Geometry check sheet. Reference: the model listing, model coordinates, mm. A direction names the side the tool comes from. Coordinates: 2 decimals unless noted, no trailing zeros. Loops run counter-clockwise (first coordinate to the right, second up) from the corner with the lowest first, then second, coordinate; pieces in that order, holes last. Notation, with made-up numbers: (83, -16) -> (89, -16) arc R6 cw to (89, -8) -> close; hole circle Ø1 at (36.25, 1). An arc over 180 degrees is marked (long way). Answer as a JSON object with one key per item and string values.
from build123d import *

# Parameters (mm, degrees)
SKETCH_1_W                = 60
SKETCH_1_H                = 60
SKETCH_1_W_2              = 50
SKETCH_1_H_2              = 50
EXTRUDE_1_DEPTH           = 84
EXTRUDE_2_DEPTH           = 34
EXTRUDE_5_DEPTH           = 34
EXTRUDE_6_DEPTH           = 34
EXTRUDE_7_DEPTH           = 34
SKETCH_12_R               = 36.5
EXTRUDE_8_DEPTH           = 5
EXTRUDE_START             = -5
SKETCH_13_R               = 36.5
EXTRUDE_9_DEPTH           = 5
SKETCH_14_R               = 36.5
EXTRUDE_10_DEPTH          = 5
SKETCH_15_R               = 36.5
EXTRUDE_11_DEPTH          = 5
SKETCH_22_W               = 29
SKETCH_22_H               = 28.5
SKETCH_22_W_2             = 28.5
SKETCH_22_H_2             = 29
EXTRUDE_12_DEPTH          = 60
SKETCH_18_R               = 1.45
CUT_EXTRUDE_2_DEPTH       = 5
PATTERN_CIRCULAR_1_COUNT  = 8
SKETCH_19_R               = 1.45
CUT_EXTRUDE_3_DEPTH       = 5
PATTERN_CIRCULAR_2_COUNT  = 8
CUT_EXTRUDE_START         = -5
SKETCH_20_R               = 1.45
CUT_EXTRUDE_4_DEPTH       = 5
PATTERN_CIRCULAR_3_COUNT  = 8
SKETCH_21_R               = 1.45
CUT_EXTRUDE_5_DEPTH       = 5
PATTERN_CIRCULAR_4_COUNT  = 8
SKETCH_26_W               = 34
SKETCH_26_H               = 28.5
SKETCH_26_W_2             = 28.5
SKETCH_26_H_2             = 34
CUT_EXTRUDE_7_DEPTH       = 58.75
SKETCH_27_R               = 10.5
CUT_EXTRUDE_8_DEPTH       = 200
SKETCH_28_R               = 10.5
CUT_EXTRUDE_9_DEPTH       = 200
SKETCH_31_R               = 2.4
CUT_EXTRUDE_12_DEPTH      = 200
SKETCH_32_R               = 2.4
CUT_EXTRUDE_13_DEPTH      = 200
CUT_EXTRUDE_14_DEPTH      = 50
CUT_EXTRUDE_14_DEPTH_BACK = 40
SKETCH_33_W               = 11
SKETCH_33_H               = 10
CUT_EXTRUDE_15_DEPTH      = 60
CUT_EXTRUDE_15_DEPTH_BACK = 40
SKETCH_34_W               = 10
SKETCH_34_H               = 11
SKETCH_35_W               = 11
SKETCH_35_H               = 10
CUT_EXTRUDE_16_DEPTH      = 80
SKETCH_36_W               = 10
SKETCH_36_H               = 11
CUT_EXTRUDE_17_DEPTH      = 80


with BuildPart() as part:
    # 草图1 → 拉伸-薄壁1 (new body)
    with BuildSketch(Plane.XY):
        with Locations((-65.869565217, 24.858695652)):
            Rectangle(SKETCH_1_W, SKETCH_1_H)
        with Locations((-65.869565217, 24.858695652)):
            Rectangle(SKETCH_1_W_2, SKETCH_1_H_2, mode=Mode.SUBTRACT)
    extrude(amount=EXTRUDE_1_DEPTH)

    # 草图5 → 凸台-拉伸2 (add)
    with BuildSketch(Plane(origin=(-35.869565217, 0, 0), x_dir=(0, 0, -1), z_dir=(1, 0, 0))):
        Polygon((0, 54.858695652), (-5, 54.858695652), (-84, 54.858695652), (-84, 39.108695652), (-5, 39.108695652), (-5, 10.608695652), (-84, 10.608695652), (-84, -5.141304348), (-5, -5.141304348), (0, -5.141304348), align=None)
    extrude(amount=EXTRUDE_2_DEPTH)

    # 草图8 → 凸台-拉伸5 (add)
    with BuildSketch(Plane(origin=(0, 54.858695652, 0), x_dir=(1, 0, 0), z_dir=(0, 1, 0))):
        Polygon((-95.869565217, 0), (-35.869565217, 0), (-35.869565217, -5), (-35.869565217, -84), (-51.619565217, -84), (-51.619565217, -5), (-80.119565217, -5), (-80.119565217, -84), (-95.869565217, -84), (-95.869565217, -5), align=None)
    extrude(amount=EXTRUDE_5_DEPTH)

    # 草图9 → 凸台-拉伸6 (add)
    with BuildSketch(Plane.ZY.offset(95.869565217)):
        Polygon((0, -5.141304348), (5, -5.141304348), (84, -5.141304348), (84, 10.608695652), (5, 10.608695652), (5, 39.108695652), (84, 39.108695652), (84, 54.858695652), (5, 54.858695652), (0, 54.858695652), align=None)
    extrude(amount=EXTRUDE_6_DEPTH)

    # 草图10 → 凸台-拉伸7 (add)
    with BuildSketch(Plane(origin=(0, -5.141304348, 0), x_dir=(-1, 0, 0), z_dir=(0, -1, 0))):
        Polygon((95.869565217, 0), (35.869565217, 0), (35.869565217, -6.658214143), (35.869565217, -84), (51.619565217, -84), (51.619565217, -6.658214143), (80.119565217, -6.658214143), (80.119565217, -84), (95.869565217, -84), (95.869565217, -6.658214143), align=None)
    extrude(amount=EXTRUDE_7_DEPTH)

    # 草图12 → 凸台-拉伸8 (add)
    with BuildSketch(Plane.ZY.offset(129.869565217)):
        with Locations((36.5, 24.858695652)):
            Circle(SKETCH_12_R)
    extrude(amount=-EXTRUDE_8_DEPTH)

    # 草图13 → 凸台-拉伸9 (add)
    with BuildSketch(Plane(origin=(-1.869565217, 0, 0), x_dir=(0, 0, -1), z_dir=(1, 0, 0)).offset(EXTRUDE_START)):
        with Locations((-36.5, 24.858695652)):
            Circle(SKETCH_13_R)
    extrude(amount=EXTRUDE_9_DEPTH)

    # 草图14 → 凸台-拉伸10 (add)
    with BuildSketch(Plane(origin=(0, 88.858695652, 0), x_dir=(1, 0, 0), z_dir=(0, 1, 0))):
        with Locations((-65.869565217, -36.5)):
            Circle(SKETCH_14_R)
    extrude(amount=-EXTRUDE_10_DEPTH)

    # 草图15 → 凸台-拉伸11 (add)
    with BuildSketch(Plane(origin=(0, -39.141304348, 0), x_dir=(-1, 0, 0), z_dir=(0, -1, 0)).offset(EXTRUDE_START)):
        with Locations((65.869565217, -36.5)):
            Circle(SKETCH_15_R)
    extrude(amount=EXTRUDE_11_DEPTH)

    # 草图22 → 凸台-拉伸12 (add)
    with BuildSketch(Plane.XY.offset(5)):
        with Locations((-110.369565217, 24.858695652)):
            Rectangle(SKETCH_22_W, SKETCH_22_H)
        with Locations((-65.869565217, 69.358695652)):
            Rectangle(SKETCH_22_W_2, SKETCH_22_H_2)
        with Locations((-21.369565217, 24.858695652)):
            Rectangle(SKETCH_22_W, SKETCH_22_H)
        with Locations((-65.869565217, -19.641304348)):
            Rectangle(SKETCH_22_W_2, SKETCH_22_H_2)
    extrude(amount=EXTRUDE_12_DEPTH)

    # 草图18 → 切除-拉伸2 (cut)
    with BuildSketch(Plane(origin=(0, 88.858695652, 0), x_dir=(1, 0, 0), z_dir=(0, 1, 0))):
        with Locations(Location((-98.369565217, -36.5, 0), (0, 0, 270))):
            Circle(SKETCH_18_R)
    cut_extrude_2 = extrude(amount=-CUT_EXTRUDE_2_DEPTH, mode=Mode.SUBTRACT)

    # 阵列(圆周)1: 切除-拉伸2 ×8 about axis
    pattern_circular_1_axis = Axis((-65.869565217, 0, 36.5), (0, 1, 0))
    for i in range(1, PATTERN_CIRCULAR_1_COUNT):
        add(cut_extrude_2.rotate(pattern_circular_1_axis, i * 360 / PATTERN_CIRCULAR_1_COUNT), mode=Mode.SUBTRACT)

    # 草图19 → 切除-拉伸3 (cut)
    with BuildSketch(Plane(origin=(-1.869565217, 0, 0), x_dir=(0, 0, -1), z_dir=(1, 0, 0))):
        with Locations(Location((-36.5, 57.358695652, 0), (0, 0, 90))):
            Circle(SKETCH_19_R)
    cut_extrude_3 = extrude(amount=-CUT_EXTRUDE_3_DEPTH, mode=Mode.SUBTRACT)

    # 阵列(圆周)2: 切除-拉伸3 ×8 about axis
    pattern_circular_2_axis = Axis((0, 24.858695652, 36.5), (1, 0, 0))
    for i in range(1, PATTERN_CIRCULAR_2_COUNT):
        add(cut_extrude_3.rotate(pattern_circular_2_axis, i * 360 / PATTERN_CIRCULAR_2_COUNT), mode=Mode.SUBTRACT)

    # 草图20 → 切除-拉伸4 (cut)
    with BuildSketch(Plane(origin=(0, -39.141304348, 0), x_dir=(-1, 0, 0), z_dir=(0, -1, 0)).offset(CUT_EXTRUDE_START)):
        with Locations(Location((98.369565217, -36.5, 0), (0, 0, 270))):
            Circle(SKETCH_20_R)
    cut_extrude_4 = extrude(amount=CUT_EXTRUDE_4_DEPTH, mode=Mode.SUBTRACT)

    # 阵列(圆周)3: 切除-拉伸4 ×8 about axis
    pattern_circular_3_axis = Axis((-65.869565217, 0, 36.5), (0, 1, 0))
    for i in range(1, PATTERN_CIRCULAR_3_COUNT):
        add(cut_extrude_4.rotate(pattern_circular_3_axis, i * 360 / PATTERN_CIRCULAR_3_COUNT), mode=Mode.SUBTRACT)

    # 草图21 → 切除-拉伸5 (cut)
    with BuildSketch(Plane.ZY.offset(129.869565217).offset(CUT_EXTRUDE_START)):
        with Locations(Location((36.5, 57.358695652, 0), (0, 0, 90))):
            Circle(SKETCH_21_R)
    cut_extrude_5 = extrude(amount=CUT_EXTRUDE_5_DEPTH, mode=Mode.SUBTRACT)

    # 阵列(圆周)4: 切除-拉伸5 ×8 about axis
    pattern_circular_4_axis = Axis((0, 24.858695652, 36.5), (1, 0, 0))
    for i in range(1, PATTERN_CIRCULAR_4_COUNT):
        add(cut_extrude_5.rotate(pattern_circular_4_axis, i * 360 / PATTERN_CIRCULAR_4_COUNT), mode=Mode.SUBTRACT)

    # 草图26 → 切除-拉伸7 (cut)
    with BuildSketch(Plane.XY.offset(84)):
        with Locations((-112.869565217, 24.858695652)):
            Rectangle(SKETCH_26_W, SKETCH_26_H)
        with Locations((-65.869565217, 71.858695652)):
            Rectangle(SKETCH_26_W_2, SKETCH_26_H_2)
        with Locations((-18.869565217, 24.858695652)):
            Rectangle(SKETCH_26_W, SKETCH_26_H)
        with Locations((-65.869565217, -22.141304348)):
            Rectangle(SKETCH_26_W_2, SKETCH_26_H_2)
    extrude(amount=-CUT_EXTRUDE_7_DEPTH, mode=Mode.SUBTRACT)

    # 草图27 → 切除-拉伸8 (cut)
    with BuildSketch(Plane.ZY.offset(129.869565217)):
        with Locations((36.5, 24.858695652)):
            Circle(SKETCH_27_R)
    extrude(amount=-CUT_EXTRUDE_8_DEPTH, mode=Mode.SUBTRACT)

    # 草图28 → 切除-拉伸9 (cut)
    with BuildSketch(Plane(origin=(0, 88.858695652, 0), x_dir=(1, 0, 0), z_dir=(0, 1, 0))):
        with Locations(Location((-65.869565217, -36.5, 0), (0, 0, 270))):
            Circle(SKETCH_28_R)
    extrude(amount=-CUT_EXTRUDE_9_DEPTH, mode=Mode.SUBTRACT)

    # 草图31 → 切除-拉伸12 (cut)
    with BuildSketch(Plane.ZY.offset(95.869565217)):
        with Locations((28.5, 13.858695652)):
            Circle(SKETCH_31_R)
        with Locations((28.5, 35.858695652)):
            Circle(SKETCH_31_R)
        with Locations((68.5, 35.858695652)):
            Circle(SKETCH_31_R)
        with Locations((68.5, 13.858695652)):
            Circle(SKETCH_31_R)
    extrude(amount=-CUT_EXTRUDE_12_DEPTH, mode=Mode.SUBTRACT)

    # 草图32 → 切除-拉伸13 (cut)
    with BuildSketch(Plane(origin=(0, -5.141304348, 0), x_dir=(-1, 0, 0), z_dir=(0, -1, 0))):
        with Locations(Location((76.869565217, -28.5, 0), (0, 0, 90))):
            Circle(SKETCH_32_R)
        with Locations(Location((54.869565217, -28.5, 0), (0, 0, 90))):
            Circle(SKETCH_32_R)
        with Locations(Location((54.869565217, -68.5, 0), (0, 0, 90))):
            Circle(SKETCH_32_R)
        with Locations(Location((76.869565217, -68.5, 0), (0, 0, 90))):
            Circle(SKETCH_32_R)
    extrude(amount=-CUT_EXTRUDE_13_DEPTH, mode=Mode.SUBTRACT)

    # 草图33 → 切除-拉伸14 (cut, two sides: drawn at the far end of the back side and taken through both)
    with BuildSketch(Plane.ZY.offset(51.619565217).offset(-CUT_EXTRUDE_14_DEPTH_BACK)):
        with Locations((50.75, -10.141304348)):
            Rectangle(SKETCH_33_W, SKETCH_33_H)
    extrude(amount=CUT_EXTRUDE_14_DEPTH + CUT_EXTRUDE_14_DEPTH_BACK, mode=Mode.SUBTRACT)

    # 草图34 → 切除-拉伸15 (cut, two sides: drawn at the far end of the back side and taken through both)
    with BuildSketch(Plane(origin=(0, 10.608695652, 0), x_dir=(1, 0, 0), z_dir=(0, 1, 0)).offset(-CUT_EXTRUDE_15_DEPTH_BACK)):
        with Locations((-100.869565217, -50.75)):
            Rectangle(SKETCH_34_W, SKETCH_34_H)
    extrude(amount=CUT_EXTRUDE_15_DEPTH + CUT_EXTRUDE_15_DEPTH_BACK, mode=Mode.SUBTRACT)

    # 草图35 → 切除-拉伸16 (cut)
    with BuildSketch(Plane.ZY.offset(95.869565217)):
        with Locations((50.75, 59.858695652)):
            Rectangle(SKETCH_35_W, SKETCH_35_H)
    extrude(amount=-CUT_EXTRUDE_16_DEPTH, mode=Mode.SUBTRACT)

    # 草图36 → 切除-拉伸17 (cut)
    with BuildSketch(Plane(origin=(0, 54.858695652, 0), x_dir=(1, 0, 0), z_dir=(0, 1, 0))):
        with Locations((-30.869565217, -50.75)):
            Rectangle(SKETCH_36_W, SKETCH_36_H)
    extrude(amount=-CUT_EXTRUDE_17_DEPTH, mode=Mode.SUBTRACT)


solid = part.part
1. Depth check by flat-ended pin: P1, Ø2, axis at x = -62, y = 2, coming from the +Z side; P2, Ø8.5, axis at x = -61.5, y = -14.5, coming from the +Z side; P3, Ø1.7, axis at x = -42.89, z = 13.52, coming from the +Y side; P4, Ø1.5, axis at y = -21.5, z = 44.5, coming from the -X side. Enter the tip coordinate at first touch or a pass-through.
Evaluation:
{"P1": "passes through", "P2": "stops at z = 25.25", "P3": "stops at y = 83.86", "P4": "stops at x = -95.87"}
2. Thickness scan on probe 1 along Y at (x, z) = (-99, 45); probe 2 along X at (y, z) = (47.5, 24.5); probe 3 along Y at (x, z) = (-42, 40). Record the ranges inside material, lowest first. Write a range as from..to.
Evaluation:
{"probe 1": "y = -39.14..-34.14, -5.14..10.61, 39.11..54.86, 83.86..88.86", "probe 2": "x = -129.87..-90.87, -40.87..-1.87", "probe 3": "y = -39.14..-0.14, 49.86..88.86"}
3. Section check A-A, the plane x = -50. Record the boundary of the cut face in (y, z).
Evaluation:
{"outline": "(-39.14, 0) -> (-0.14, 0) -> (-0.14, 84) -> (-39.14, 84) -> close; (49.86, 0) -> (88.86, 0) -> (88.86, 84) -> (49.86, 84) -> close; hole (-15.14, 45.25) -> (-5.14, 45.25) -> (-5.14, 56.25) -> (-15.14, 56.25) -> close; hole (54.86, 45.25) -> (64.86, 45.25) -> (64.86, 56.25) -> (54.86, 56.25) -> close"}
4. Section check B-B, the plane y = -13.5. Record the boundary of the cut face in (x, z).
Evaluation:
{"outline": "(-95.87, 0) -> (-35.87, 0) -> (-35.87, 45.25) -> (-51.62, 45.25) -> (-51.62, 25.25) -> (-80.12, 25.25) -> (-80.12, 45.25) -> (-95.87, 45.25) -> close; (-95.87, 56.25) -> (-80.12, 56.25) -> (-80.12, 84) -> (-95.87, 84) -> close; (-51.62, 56.25) -> (-35.87, 56.25) -> (-35.87, 84) -> (-51.62, 84) -> close"}
5. Tool access check on faces 5 (the face through (-19, 39.109, 55)), 6 (the face through (-31, 47, 45.25)), 7 (the face through (-29.37, 86.39, 36.81)). Record the directions out of +Z, -Z, +X, -X, +Y, -Y that give a thin tool (end or side, any length) a straight path to the whole face; none if there is none.
Evaluation:
{"face 5": "+Z, +X", "face 6": "none", "face 7": "+X, +Y"}
6. Section check D-D, the plane y = 31. Record the boundary of the cut face in (x, z), then the cut area to 3 significant figures.
Evaluation:
{"outline": "(-129.87, 0) -> (-90.87, 0) -> (-90.87, 27.98) -> (-95.87, 27.98) -> (-95.87, 25.25) -> (-129.87, 25.25) -> close; (-95.87, 45.02) -> (-90.87, 45.02) -> (-90.87, 84) -> (-95.87, 84) -> close; (-40.87, 0) -> (-1.87, 0) -> (-1.87, 25.25) -> (-35.87, 25.25) -> (-35.87, 27.98) -> (-40.87, 27.98) -> close; (-40.87, 45.02) -> (-35.87, 45.02) -> (-35.87, 84) -> (-40.87, 84) -> close", "area": "2,390 mm^2"}
7. Mould release check, pull along Z, two halves, no side actions. Record for faces 1 (the face through (-90.87, 25, 51)), 2 (the face through (-127.405, 61.357, 36.81)), 3 (the face through (-93, 25, 26)), 4 (the face through (-44, 60, 45.25)): released by +Z, released by -Z, zero draft, split by the parting line, or undercut.
Evaluation:
{"face 1": "zero draft", "face 2": "split by the parting line", "face 3": "undercut", "face 4": "undercut"}
